Can you work these out from the model? Positions are in its coordinate system, mm. Face numbers are marked on the shaded views. A direction names the side the tool comes from. Give positions to 0.01 mm unless a question says otherwise; leave off trailing zeros. Order: outer loops, then holes, each group sorted by start corner. A loop starts at its lowest first (then second) coordinate and runs counter-clockwise, first axis right, second up. Notation, with made-up numbers: (27, -28.75) - (78, -28.75) arc R35 cw to (78, 10.25) - close; hole circle Ø5 at (38.5, -19). An arc over 180 degrees is marked (long way). Write each question's results on one line, items separated by ' | '. Start each with the question number.
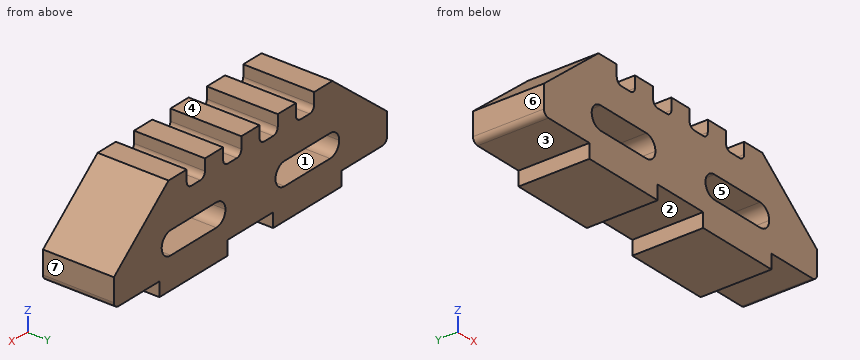
from build123d import *

# Parameters (mm, degrees)
F1_DEPTH = 25


with BuildPart() as f1:
    # F0 (on Front) → F1 (new body)
    with BuildSketch(Plane.XZ):
        with BuildLine():
            ThreePointArc((-225.4685461521, -62.0369579196), (-224.8827597145, -63.451171482), (-223.4685461521, -64.0369579196))
            Line((-223.4685461521, -64.0369579196), (-205.4685461521, -64.0369579196))
            Line((-205.4685461521, -64.0369579196), (-205.4685461521, -69.0369579196))
            Line((-205.4685461521, -69.0369579196), (-175.4685461521, -69.0369579196))
            Line((-175.4685461521, -69.0369579196), (-175.4685461521, -64.0369579196))
            Line((-175.4685461521, -64.0369579196), (-165.4685461521, -64.0369579196))
            Line((-165.4685461521, -64.0369579196), (-165.4685461521, -54.0369579196))
            Line((-165.4685461521, -54.0369579196), (-165.4685461521, -34.0369579196))
            Line((-165.4685461521, -34.0369579196), (-169.4685461521, -34.0369579196))
            Line((-169.4685461521, -34.0369579196), (-169.4685461521, -38.0369579196))
            ThreePointArc((-169.4685461521, -38.0369579196), (-170.0543325897, -39.451171482), (-171.4685461521, -40.0369579196))
            Line((-171.4685461521, -40.0369579196), (-175.4685461521, -40.0369579196))
            ThreePointArc((-175.4685461521, -40.0369579196), (-176.8827597145, -39.451171482), (-177.4685461521, -38.0369579196))
            Line((-177.4685461521, -38.0369579196), (-177.4685461521, -34.0369579196))
            Line((-177.4685461521, -34.0369579196), (-185.4685461521, -34.0369579196))
            Line((-185.4685461521, -34.0369579196), (-185.4685461521, -38.0369579196))
            ThreePointArc((-185.4685461521, -38.0369579196), (-186.0543325897, -39.451171482), (-187.4685461521, -40.0369579196))
            Line((-187.4685461521, -40.0369579196), (-191.4685461521, -40.0369579196))
            ThreePointArc((-191.4685461521, -40.0369579196), (-192.8827597145, -39.451171482), (-193.4685461521, -38.0369579196))
            Line((-193.4685461521, -38.0369579196), (-193.4685461521, -34.0369579196))
            Line((-193.4685461521, -34.0369579196), (-201.4685461521, -34.0369579196))
            Line((-201.4685461521, -34.0369579196), (-225.4685461521, -54.0369579196))
            Line((-225.4685461521, -54.0369579196), (-225.4685461521, -62.0369579196))
        make_face()
        with BuildLine():
            ThreePointArc((-180.4685461521, -50.0369579196), (-177.6401190274, -51.2085307949), (-176.4685461521, -54.0369579196))
            ThreePointArc((-176.4685461521, -54.0369579196), (-177.6401190274, -56.8653850443), (-180.4685461521, -58.0369579196))
            Line((-180.4685461521, -58.0369579196), (-200.4685461521, -58.0369579196))
            ThreePointArc((-200.4685461521, -58.0369579196), (-203.2969732769, -56.8653850443), (-204.4685461521, -54.0369579196))
            ThreePointArc((-204.4685461521, -54.0369579196), (-203.2969732769, -51.2085307949), (-200.4685461521, -50.0369579196))
            Line((-200.4685461521, -50.0369579196), (-180.4685461521, -50.0369579196))
        make_face(mode=Mode.SUBTRACT)
        with BuildLine():
            Line((-165.4685461521, -34.0369579196), (-165.4685461521, -54.0369579196))
            Line((-165.4685461521, -54.0369579196), (-154.4685461521, -54.0369579196))
            ThreePointArc((-154.4685461521, -54.0369579196), (-153.2969732769, -51.2085307949), (-150.4685461521, -50.0369579196))
            Line((-150.4685461521, -50.0369579196), (-130.4685461521, -50.0369579196))
            ThreePointArc((-130.4685461521, -50.0369579196), (-127.6401190274, -51.2085307949), (-126.4685461521, -54.0369579196))
            ThreePointArc((-126.4685461521, -54.0369579196), (-127.6401190274, -56.8653850443), (-130.4685461521, -58.0369579196))
            Line((-130.4685461521, -58.0369579196), (-140.4685461521, -58.0369579196))
            Line((-140.4685461521, -58.0369579196), (-140.4685461521, -69.0369579196))
            Line((-140.4685461521, -69.0369579196), (-125.4685461521, -69.0369579196))
            Line((-125.4685461521, -69.0369579196), (-125.4685461521, -64.0369579196))
            Line((-125.4685461521, -64.0369579196), (-107.4685461521, -64.0369579196))
            ThreePointArc((-107.4685461521, -64.0369579196), (-106.0543325897, -63.451171482), (-105.4685461521, -62.0369579196))
            Line((-105.4685461521, -62.0369579196), (-105.4685461521, -54.0369579196))
            Line((-105.4685461521, -54.0369579196), (-129.4685461521, -34.0369579196))
            Line((-129.4685461521, -34.0369579196), (-137.4685461521, -34.0369579196))
            Line((-137.4685461521, -34.0369579196), (-137.4685461521, -38.0369579196))
            ThreePointArc((-137.4685461521, -38.0369579196), (-138.0543325897, -39.451171482), (-139.4685461521, -40.0369579196))
            Line((-139.4685461521, -40.0369579196), (-143.4685461521, -40.0369579196))
            ThreePointArc((-143.4685461521, -40.0369579196), (-144.8827597145, -39.451171482), (-145.4685461521, -38.0369579196))
            Line((-145.4685461521, -38.0369579196), (-145.4685461521, -34.0369579196))
            Line((-145.4685461521, -34.0369579196), (-153.4685461521, -34.0369579196))
            Line((-153.4685461521, -34.0369579196), (-153.4685461521, -38.0369579196))
            ThreePointArc((-153.4685461521, -38.0369579196), (-154.0543325897, -39.451171482), (-155.4685461521, -40.0369579196))
            Line((-155.4685461521, -40.0369579196), (-159.4685461521, -40.0369579196))
            ThreePointArc((-159.4685461521, -40.0369579196), (-160.8827597145, -39.451171482), (-161.4685461521, -38.0369579196))
            Line((-161.4685461521, -38.0369579196), (-161.4685461521, -34.0369579196))
            Line((-161.4685461521, -34.0369579196), (-165.4685461521, -34.0369579196))
        make_face()
        with BuildLine():
            Line((-165.4685461521, -54.0369579196), (-165.4685461521, -64.0369579196))
            Line((-165.4685461521, -64.0369579196), (-155.4685461521, -64.0369579196))
            Line((-155.4685461521, -64.0369579196), (-155.4685461521, -69.0369579196))
            Line((-155.4685461521, -69.0369579196), (-140.4685461521, -69.0369579196))
            Line((-140.4685461521, -69.0369579196), (-140.4685461521, -58.0369579196))
            Line((-140.4685461521, -58.0369579196), (-150.4685461521, -58.0369579196))
            ThreePointArc((-150.4685461521, -58.0369579196), (-153.2969732769, -56.8653850443), (-154.4685461521, -54.0369579196))
            Line((-154.4685461521, -54.0369579196), (-165.4685461521, -54.0369579196))
        make_face()
    extrude(amount=F1_DEPTH)


solid = f1.part
Q1. If we section it at A-A (x = -198): Please give me the cut outline in (y, z).
Q2. Will these pins go through, and if not, where does the flat tip stop? P1, Ø4, axis at y = -10, z = -66.5, coming from the +X side; P2, Ø3, axis at y = -10, z = -36.5, coming from the +X side; P3, Ø1.2, axis at y = -7.5, z = -36.5, coming from the -X side.
Q3. If we section it at C-C (y = -16): State how many separate pieces and enclosed holes the cut face has, plus the area to 3 significant figures.
Q4. If I drill on probe 1 along Z at (x, y) = (-196.5, -18); probe 2 along X at (y, z) = (-6.25, -55); probe 3 along X at (y, z) = (-24, -38.5), over which ranges is the centre line in solid material (lowest first)? Write a range as from..to.
Q5. If we section it at D-D (x = -211): Please give me the cut outline in (y, z).
Q6. If we section it at B-B (z = -56.5): Please give me the cut outline in (x, y).
Q7. Thinking about a two-plate mould opening in X: for the marked faces 4, 5, 6 and 7, which applies, released by +X, released by -X, zero draft, split by the parting line, or undercut?
Q8. Which directions (+Z, -Z, +X, -X, +Y, -Y) give clear straight access to the entire face, cutting with the end or side of a thin tool? Please do the marked faces 1, 2 and 3.
Findings below:
1) outline: (-25, -69.04) - (0, -69.04) - (0, -58.04) - (-25, -58.04) - close; (-25, -50.04) - (0, -50.04) - (0, -34.04) - (-25, -34.04) - close
2) P1: stops at x = -125.47 | P2: stops at x = -124.71 | P3: stops at x = -205.14
3) separate pieces: 1 | enclosed holes: 2 | area: 2,810 mm2
4) probe 1: z = -69.04..-58.04, -50.04..-34.04 | probe 2: x = -225.47..-204.35, -176.59..-154.35, -126.59..-105.47 | probe 3: x = -206.82..-193.41, -185.52..-177.41, -169.52..-161.41, -153.52..-145.41, -137.52..-124.11
5) outline: (-25, -64.04) - (0, -64.04) - (0, -41.98) - (-25, -41.98) - close
6) outline: (-225.47, -25) - (-203.62, -25) - (-203.62, 0) - (-225.47, 0) - close; (-177.32, -25) - (-153.62, -25) - (-153.62, 0) - (-177.32, 0) - close; (-127.32, -25) - (-105.47, -25) - (-105.47, 0) - (-127.32, 0) - close
7) face 4: zero draft | face 5: undercut | face 6: released by -X | face 7: released by +X
8) face 1: +Y, -Y | face 2: -Z, +Y, -Y | face 3: -Z, -X, +Y, -Y
